Source: CAD feature listing. Evaluate the final solid. Frame: model axes, mm. Face numbers are marked on the shaded views. A direction names the side the tool comes from. Coordinates: 2 decimals unless noted, no trailing zeros. Order: outer loops, then holes, each group sorted by start corner. A loop starts at its lowest first (then second) coordinate and runs counter-clockwise, first axis right, second up. Notation, with made-up numbers: (66.25, 2) -> (117.25, 2) arc R14 ccw to (117.25, 9) -> close; hole circle Ø4 at (-14, 49.5). An arc over 180 degrees is marked (long way). Write item = value, one per line. Start each with the question number.
Item 1: Mould query, pull axis X, two halves, no side actions, for the marked faces 1, 2, 3 and 4. Classes: released by +X, released by -X, zero draft, split by the parting line, or undercut.
Item 2: Ray query, line 1 along X through (y, z) = (12, 1). Return the intervals inside material, ascending. Write a range as [from, to].
Item 3: Section query B-B (z = -5). Output: boundary loops of the cut face in (x, y), then the cut area to 3 significant figures.
Item 4: Section query A-A (x = -17.5). Output: boundary loops of the cut face in (y, z).
Item 5: Set-up query: the marked faces 5 and 6. Return all of +Z, -Z, +X, -X, +Y, -Y with unobstructed straight access to the full face (end or side cutting, diameter ignored); none if empty.
Item 6: Section query C-C (y = 42). Output: boundary loops of the cut face in (x, z), then the cut area to 3 significant figures.
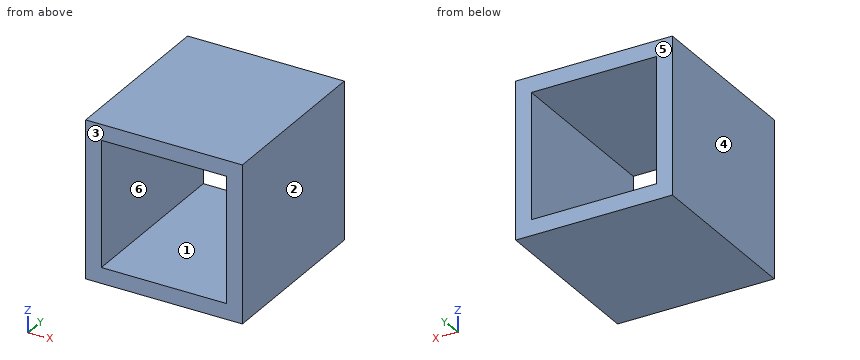
Autodesk Inventor part; units mm, degrees
ref_plane "YZ Plane" through (0, 0, 0) normal (1, 0, 0) x (0, 1, 0)
ref_plane "XZ Plane" through (0, 0, 0) normal (0, 1, 0) x (-1, 0, 0)
ref_plane "XY Plane" through (0, 0, 0) normal (0, 0, 1) x (1, 0, 0)
sketch "Sketch1" plane through (0, 0, 0) normal (0, 1, 0) x (-1, 0, 0)
  line L0 (50, -50) -> (-50, -50)
  line L1 (-50, -50) -> (-50, 50)
  line L2 (-50, 50) -> (50, 50)
  line L3 (50, 50) -> (50, -50)
  line L4 (50, -50) -> (-50, 50) construction
  line L5 (-50, -50) -> (50, 50) construction
  line L6 (-40, -40) -> (40, -40)
  line L7 (40, -40) -> (40, 40)
  line L8 (40, 40) -> (-40, 40)
  line L9 (-40, 40) -> (-40, -40)
  line L10 (-40, -40) -> (40, 40) construction
  line L11 (40, -40) -> (-40, 40) construction
  point P0 (0, 0)
  dimension "d0" = 100
  dimension "d1" = 100
  dimension "d2" = 80
  dimension "d3" = 80
extrude "Extrusion1" add sketch "Sketch1" along normal blind 110
properties part number "D1_lenght" material "Steel, Alloy"
Computed:
q1.face_1 = undercut
q1.face_2 = released by +X
q1.face_3 = zero draft
q1.face_4 = released by -X
q2.line_1 = [-50, -40], [40, 50]
q3.outline = (-50, 0) -> (-40, 0) -> (-40, 110) -> (-50, 110) -> close; (40, 0) -> (50, 0) -> (50, 110) -> (40, 110) -> close
q3.area = 2,200 mm^2
q4.outline = (0, -50) -> (110, -50) -> (110, -40) -> (0, -40) -> close; (0, 40) -> (110, 40) -> (110, 50) -> (0, 50) -> close
q5.face_5 = +Z, -Z, +X, -X, +Y
q5.face_6 = +Y, -Y
q6.outline = (-50, -50) -> (50, -50) -> (50, 50) -> (-50, 50) -> close; hole (-40, -40) -> (40, -40) -> (40, 40) -> (-40, 40) -> close
q6.area = 3,600 mm^2
